from build123d import *

# Parameters (mm, degrees)
SKETCH_1_W      = 23
SKETCH_1_H      = 12
EXTRUDE_1_DEPTH = 20
SKETCH_2_W      = 4
SKETCH_2_H      = 12
SKETCH_2_R      = 1.5
EXTRUDE_2_DEPTH = 2
SKETCH_3_W      = 23
SKETCH_3_H      = 12
EXTRUDE_3_DEPTH = 4
SKETCH_4_R      = 2.5
EXTRUDE_4_DEPTH = 5


with BuildPart() as part:
    # 草图1 → 凸台-拉伸1 (new body)
    with BuildSketch(Plane.XY):
        with Locations((11.5, 6)):
            Rectangle(SKETCH_1_W, SKETCH_1_H)
    extrude(amount=EXTRUDE_1_DEPTH)

    # 草图2 → 凸台-拉伸2 (add)
    # profile 1 of 2: a face of its own
    with BuildSketch(Plane.XY.offset(20)):
        with Locations((-2, 6)):
            Rectangle(SKETCH_2_W, SKETCH_2_H)
        with Locations((-2.25, 6)):
            Circle(SKETCH_2_R, mode=Mode.SUBTRACT)
    # profile 2 of 2: a face of its own
    with BuildSketch(Plane.XY.offset(20)):
        with Locations((25, 6)):
            Rectangle(SKETCH_2_W, SKETCH_2_H)
        with Locations((25.25, 6)):
            Circle(SKETCH_2_R, mode=Mode.SUBTRACT)
    extrude(amount=-EXTRUDE_2_DEPTH)

    # 草图3 → 凸台-拉伸3 (add)
    with BuildSketch(Plane.XY.offset(20)):
        with Locations((11.5, 6)):
            Rectangle(SKETCH_3_W, SKETCH_3_H)
    extrude(amount=EXTRUDE_3_DEPTH)

    # 草图4 → 凸台-拉伸4 (add)
    with BuildSketch(Plane.XY.offset(24)):
        with Locations(Location((18.623805867, 6, 0), (0, 0, 180))):
            Circle(SKETCH_4_R)
    extrude(amount=EXTRUDE_4_DEPTH)


solid = part.part
Here's how the part is built. I have some questions about the finished solid (model axes, mm). A direction names the side the tool comes from. Give positions to 0.01 mm unless a question says otherwise; leave off trailing zeros. Loops run counter-clockwise (first coordinate to the right, second up) from the corner with the lowest first, then second, coordinate; pieces in that order, holes last. Notation, with made-up numbers: (1.25, -17) -> (29.25, -17) arc R18 cw to (29.25, -6) -> close; hole circle Ø9 at (30, -34.75). An arc over 180 degrees is marked (long way). Answer as a JSON object with one key per item and string values. Group by question number.
Item 1: Imagine slicing it at A-A on y = 6. Write out the boundary of the cut face in (x, z).
Item 2: Imagine slicing it at D-D on z = 7.5. Write out the boundary of the cut face in (x, y), then the cut area to 3 significant figures.
Item 3: Imagine slicing it at C-C on y = 11. Write out the boundary of the cut face in (x, z).
Item 4: I need wall thicknesses on L1, parallel to Y at x = 25.25, z = 19.55; L2, parallel to X at y = 0.75, z = 16.5; L3, parallel to Z at x = 4.5, y = 2.25. Which ranges of each line are inside material? Lowest first, please.
Item 5: Will these pins go through, and if not, where does the flat tip stop? pin 1 (2 mm diameter, centred on x = -1.5, y = 5.5, fed in from -Z); pin 2 (4.5 mm diameter, centred on x = 25.5, y = 8.5, fed in from +Z); pin 3 (1.2 mm diameter, centred on y = 6.5, z = 22, fed in from -X).
Item 6: Thinking about a two-plate mould opening in X: for faces 4 (the flat face through (19, 6, 29)), 5 (the cylindrical face through (-0.82, 6.45, 19.01)), 6 (the flat face through (0, 6, 9)), which applies, pulls with the +X half, pulls with the -X half, needs draft (parallel to the pull), parting line crosses it, or undercut?
Item 7: Imagine slicing it at B-B on x = 25.25. Write out the boundary of the cut face in (y, z), then the cut area to 3 significant figures.
Item 8: On a 3-axis mill with a long thin cutter (end or side, diameter ignored), from which of +Z, -Z, +X, -X, +Y, -Y can I reach the whole of each face in a straight line? I mean faces 1 (the cylindrical face through (20.466, 4.31, 26.465)), 2 (the flat face through (0, 6, 22)), 3 (the flat face through (23, 6, 9)). Say none if no direction works.
Answer list:
{
 "1": {"outline": "(-4, 18) -> (-3.75, 18) -> (-3.75, 20) -> (-4, 20) -> close; (-0.75, 18) -> (0, 18) -> (0, 0) -> (23, 0) -> (23, 18) -> (23.75, 18) -> (23.75, 20) -> (23, 20) -> (23, 24) -> (21.12, 24) -> (21.12, 29) -> (16.12, 29) -> (16.12, 24) -> (0, 24) -> (0, 20) -> (-0.75, 20) -> close; (26.75, 18) -> (27, 18) -> (27, 20) -> (26.75, 20) -> close"},
 "2": {"outline": "(0, 0) -> (23, 0) -> (23, 12) -> (0, 12) -> close", "area": "276 mm2"},
 "3": {"outline": "(-4, 18) -> (0, 18) -> (0, 0) -> (23, 0) -> (23, 18) -> (27, 18) -> (27, 20) -> (23, 20) -> (23, 24) -> (0, 24) -> (0, 20) -> (-4, 20) -> close"},
 "4": {"L1": "y = 0 to 4.5, 7.5 to 12", "L2": "x = 0 to 23", "L3": "z = 0 to 24"},
 "5": {"pin 1": "stops at z = 18", "pin 2": "stops at z = 20", "pin 3": "stops at x = 0"},
 "6": {"face 4": "needs draft", "face 5": "undercut", "face 6": "pulls with the -X half"},
 "7": {"outline": "(0, 18) -> (4.5, 18) -> (4.5, 20) -> (0, 20) -> close; (7.5, 18) -> (12, 18) -> (12, 20) -> (7.5, 20) -> close", "area": "18.0 mm2"},
 "8": {"face 1": "+Z", "face 2": "+Z, -X, +Y, -Y", "face 3": "-Z, +X, +Y, -Y"}
}
